For this review, take the finished solid that the model builds, in its own axes (mm). Give positions to 0.01 mm unless a question says otherwise; leave off trailing zeros. Loops run counter-clockwise (first coordinate to the right, second up) from the corner with the lowest first, then second, coordinate; pieces in that order, holes last.
```python
from build123d import *

# Parameters (mm, degrees)
F0_W     = 279.4
F0_H     = 249.174
F1_DEPTH = 28.575


with BuildPart() as f1:
    # F0 (on Top) → F1 (new body)
    with BuildSketch(Plane.XY):
        with BuildLine():
            Line((990.6, 533.4), (-990.6, 533.4))
            ThreePointArc((-990.6, 533.4), (-1044.481537, 511.081537), (-1066.8, 457.2))
            Line((-1066.8, 457.2), (-1066.8, 0))
            Line((-1066.8, 0), (-1066.8, -457.2))
            ThreePointArc((-1066.8, -457.2), (-1044.481537, -511.081537), (-990.6, -533.4))
            Line((-990.6, -533.4), (990.6, -533.4))
            ThreePointArc((990.6, -533.4), (1044.481537, -511.081537), (1066.8, -457.2))
            Line((1066.8, -457.2), (1066.8, 457.2))
            ThreePointArc((1066.8, 457.2), (1044.481537, 511.081537), (990.6, 533.4))
        make_face()
        with BuildLine():
            ThreePointArc((-508, 0), (-533.4, -25.4), (-558.8, 0))
            ThreePointArc((-558.8, 0), (-533.4, 25.4), (-508, 0))
        make_face(mode=Mode.SUBTRACT)
        Rectangle(F0_W, F0_H, mode=Mode.SUBTRACT)
    extrude(amount=F1_DEPTH)


solid = f1.part
```
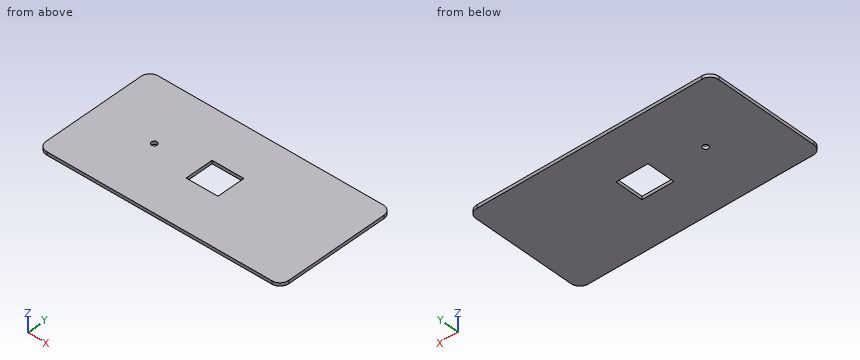
Item 1: Take a section at B-B on z = 6.75. Give the boundary of the cut face in (x, y), and give its area (3 significant figures).
Answer:
outline: (-1066.8, -457.2) arc R76.2 ccw to (-990.6, -533.4) - (990.6, -533.4) arc R76.2 ccw to (1066.8, -457.2) - (1066.8, 457.2) arc R76.2 ccw to (990.6, 533.4) - (-990.6, 533.4) arc R76.2 ccw to (-1066.8, 457.2) - close; hole circle Ø50.8 at (-533.4, 0); hole (-139.7, -124.59) - (139.7, -124.59) - (139.7, 124.59) - (-139.7, 124.59) - close
area: 2,200,000 mm2
Item 2: For L1, parallel to Y at x = -533.4, z = 19.25; L2, parallel to Y at x = 115, z = 14.5; L3, parallel to X at y = 76, z = 5.5, list the stretches that pass through material, from the lowest coordinate up.
Answer:
L1: y = -533.4 to -25.4, 25.4 to 533.4
L2: y = -533.4 to -124.59, 124.59 to 533.4
L3: x = -1066.8 to -139.7, 139.7 to 1066.8
Item 3: Take a section at A-A on y = 0. Give the boundary of the cut face in (x, z) (3 decimals).
Answer:
outline: (-1066.8, 0) - (-558.8, 0) - (-558.8, 28.575) - (-1066.8, 28.575) - close; (-508, 0) - (-139.7, 0) - (-139.7, 28.575) - (-508, 28.575) - close; (139.7, 0) - (1066.8, 0) - (1066.8, 28.575) - (139.7, 28.575) - close
Item 4: Take a section at C-C on x = -533.4. Give the boundary of the cut face in (y, z) (3 decimals), and give its area (3 significant figures).
Answer:
outline: (-533.4, 0) - (-25.4, 0) - (-25.4, 28.575) - (-533.4, 28.575) - close; (25.4, 0) - (533.4, 0) - (533.4, 28.575) - (25.4, 28.575) - close
area: 29,000 mm2
